Part model, mm, in its own coordinate system. Face numbers are marked on the shaded views. A direction names the side the tool comes from. Give positions to 0.01 mm unless a question says otherwise; leave off trailing zeros. Write each loop counter-clockwise with the first axis right and the second up, starting at its lowest first coordinate (ties: lowest second). Pieces come first, ordered by that corner, then holes.
from build123d import *

# Parameters (mm, degrees)
SKETCH1_W           = 41.91
SKETCH1_H           = 41.91
SKETCH1_R           = 1.64973
SKETCH1_R_2         = 12.7
BOSS_EXTRUDE1_DEPTH = 10.795
SKETCH3_R           = 19.84375
CUT_EXTRUDE2_DEPTH  = 7.62
CHAMFER1_SIZE       = 3.175


with BuildPart() as part:
    # Sketch1 → Boss-Extrude1 (new body)
    with BuildSketch(Plane.XY):
        with Locations((20.955, 20.955)):
            Rectangle(SKETCH1_W, SKETCH1_H)
        with Locations((37.460710751, 37.460710751)):
            Circle(SKETCH1_R, mode=Mode.SUBTRACT)
        with Locations((37.460710751, 4.449289249)):
            Circle(SKETCH1_R, mode=Mode.SUBTRACT)
        with Locations((4.449289249, 4.449289249)):
            Circle(SKETCH1_R, mode=Mode.SUBTRACT)
        with Locations((4.449289249, 37.460710751)):
            Circle(SKETCH1_R, mode=Mode.SUBTRACT)
        with Locations((20.955, 20.955)):
            Circle(SKETCH1_R_2, mode=Mode.SUBTRACT)
    extrude(amount=BOSS_EXTRUDE1_DEPTH)

    # Sketch3 → Cut-Extrude2 (cut)
    with BuildSketch(Plane.XY.offset(10.795)):
        with Locations((20.955, 20.955)):
            Circle(SKETCH3_R)
    extrude(amount=-CUT_EXTRUDE2_DEPTH, mode=Mode.SUBTRACT)

    # Chamfer1
    chamfer1_edges = [part.edges().sort_by_distance(p)[0] for p in [
        (0, 41.91, 5.3975),
        (41.91, 41.91, 5.3975),
        (41.91, 0, 5.3975),
        (0, 0, 5.3975),
    ]]
    chamfer(chamfer1_edges, length=CHAMFER1_SIZE)


solid = part.part
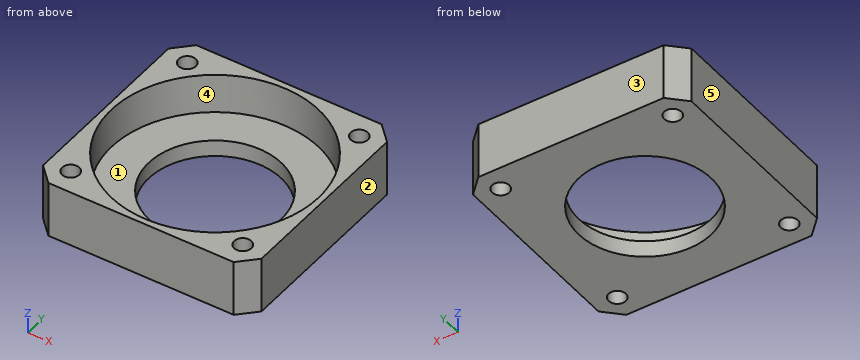
1) Mould opens along Y. For the marked faces 1, 2 and 3 say: +Y half, -Y half, draft (parallel to the pull), parting line (faces both ways), or undercut.
Check result:
face 1: undercut
face 2: draft
face 3: +Y half
2) Saw through at A-A (x = 18). Write the cut outline in (y, z) (1 decimal), and give its area (3 significant figures).
Check result:
outline: (0, 0) - (8.6, 0) - (8.6, 3.2) - (1.3, 3.2) - (1.3, 10.8) - (0, 10.8) - close; (33.3, 0) - (41.9, 0) - (41.9, 10.8) - (40.6, 10.8) - (40.6, 3.2) - (33.3, 3.2) - close
area: 74.9 mm2
3) 3-axis set-ups, long thin cutter, end or side, ignore diameter. For the marked faces 4 and 5: which of +Z, -Z, +X, -X, +Y, -Y reach the whole face in a straight line?
Check result:
face 4: +Z
face 5: +Z, -Z, -X, +Y, -Y
4) Drill centre lines: L1, parallel to X at y = 5, z = 3.5; L2, parallel to Y at x = 38, z = 4.5. Where is each one in solid material? Low to high.
Check result:
L1: x = 0 to 2.89, 6 to 9.16, 32.75 to 35.91, 39.02 to 41.91
L2: y = 0 to 2.89, 6.01 to 10.79, 31.12 to 35.9, 39.02 to 41.91
5) Saw through at D-D (x = 36.5). Write the cut outline in (y, z) (3 decimals).
Check result:
outline: (0, 0) - (3.108, 0) - (3.108, 10.795) - (0, 10.795) - close; (5.79, 0) - (36.12, 0) - (36.12, 10.795) - (33.289, 10.795) - (33.289, 3.175) - (8.621, 3.175) - (8.621, 10.795) - (5.79, 10.795) - close; (38.802, 0) - (41.91, 0) - (41.91, 10.795) - (38.802, 10.795) - close
6) Saw through at C-C (z = 8.5). Write the cut outline in (x, y) (1 decimal), and give its area (3 significant figures).
Check result:
outline: (0, 3.2) - (3.2, 0) - (38.7, 0) - (41.9, 3.2) - (41.9, 38.7) - (38.7, 41.9) - (3.2, 41.9) - (0, 38.7) - close; hole circle Ø39.7 at (21, 21); hole circle Ø3.3 at (4.4, 4.4); hole circle Ø3.3 at (4.4, 37.5); hole circle Ø3.3 at (37.5, 4.4); hole circle Ø3.3 at (37.5, 37.5)
area: 465 mm2
7) Saw through at B-B (y = 28). Write the cut outline in (x, z) (3 decimals), and give its area (3 significant figures).
Check result:
outline: (0, 0) - (10.388, 0) - (10.388, 3.175) - (2.404, 3.175) - (2.404, 10.795) - (0, 10.795) - close; (31.522, 0) - (41.91, 0) - (41.91, 10.795) - (39.506, 10.795) - (39.506, 3.175) - (31.522, 3.175) - close
area: 103 mm2
8) Flat gauge pins, fed straight in: P1, Ø5.5, axis at x = 37.46, y = 4.45, coming from the +Z side (3 decimals); P2, Ø2.5, axis at x = 4.45, y = 37.46, coming from the -Z side; P3, Ø12, axis at x = 22.5, y = 28.5, coming from the +Z side (3 decimals). Where does each tip first touch, or does it go through?
Check result:
P1: stops at z = 10.795
P2: passes through
P3: stops at z = 3.175
